Verification items for the finished model (mm, model axes). A direction names the side the tool comes from. Round coordinates to 2 decimals unless told otherwise and drop trailing zeros. Order: outer loops, then holes, each group sorted by start corner. A loop starts at its lowest first (then second) coordinate and runs counter-clockwise, first axis right, second up. Notation, with made-up numbers: M -20.75,-21 L 11.25,-21 A33 cw 11.25,8 Z; hole C -1,1.5 d4. An arc over 180 degrees is marked long. Use CSV: the item, a comma, the result in double quotes. Start each with the question number.
Q1. Sectioned sample at B-B (y = -9.5). Enter the section's corners in (x, z).
Q2. Set-up check for faces 1 (the face through (13, -15, -1.375)), 2 (the face through (13, -13.4, -4)), 3 (the face through (13, 0, 2)), 4 (the face through (-4, -3, -5)): record each of +Z, -Z, +X, -X, +Y, -Y from which the full face is reachable in a straight line by a thin tool's end or side.
Q3. Mould release check, pull along Y, two halves, no side actions. Record for faces 5 (the face through (-13.12, -14.784, -10.644)), 6 (the face through (0.195, 3.513, 11.032)), 7 (the face through (22.5, -3.8, -0.1)): +Y half, -Y half, draft (parallel to the pull), parting line (faces both ways), or undercut.
Q4. Scan lines: line 1 (X direction, y = 5, z = 10.25); line 2 (Y direction, x = -15, z = 10); line 3 (X direction, y = -3.5, z = -9). Record each from-to range of solid material in increasing order.
Q5. Gauge pin test, flat ends, axial feed: pin 1 Ø6 at (x, z) = (13, 7) entering from +Y; pin 2 Ø1.5 at (x, y) = (-7.5, -6) entering from -Z; pin 3 Ø4 at (x, y) = (15, 5) entering from -Z (3 decimals); pin 4 Ø14 at (y, z) = (-4.5, -3) entering from +X. Record the tip position at first contact, or that the pin passes through.
Q6. Sectioned sample at A-A (z = 1.5). Enter the section's corners in (x, y), and give its area (3 significant figures).
```python
from build123d import *

# Parameters (mm, degrees)
F0_W        = 45
F0_H        = 26.25
F1_DEPTH    = 17.4
F2_W        = 45
F2_H        = 4
F3_DEPTH    = 10
F5_DEPTH    = 45
F7_D        = 3
F8_T1_DEPTH = 112.5981529113
F9_W        = 8
F9_H        = 22.25
F9_H_2      = 1.1180170857
F10_DEPTH   = 21.5
F11_R       = 8.69999
F12_R       = 1


# Not quite as in the source:
# - a fillet or chamfer that OpenCascade refuses, or shapes differently, is made with other operations: its cross-section is extruded or revolved along the edge and cut away or added
# - a fillet or chamfer is up to 0.001 mm smaller than in the source, because OpenCascade refuses the exact size


with BuildPart() as f1:
    # F0 (on Front) → F1 (new body)
    with BuildSketch(Plane.XZ):
        Rectangle(F0_W, F0_H)
    extrude(amount=F1_DEPTH)

    # F2 (on face) → F3 (join)
    with BuildSketch(Plane(origin=(0, 0, 0), x_dir=(-1, 0, 0), z_dir=(0, 1, 0))):
        with Locations((0, 11.125)):
            Rectangle(F2_W, F2_H)
    extrude(amount=F3_DEPTH)

    # F4 (on face) → F5 (cut)
    with BuildSketch(Plane.YZ.offset(22.5)):
        with BuildLine():
            Line((-13.4, -1.375), (-13.4, -6.375))
            ThreePointArc((-13.4, -6.375), (-11.2118515201, -9.0669923606), (-8.1295833678, -7.475))
            Line((-8.1295833678, -7.475), (-4.5024615599, -7.475))
            Line((-4.5024615599, -7.475), (-4, -7.475))
            Line((-4, -7.475), (-4, 13.125))
            Line((-4, 13.125), (-17.4, 13.125))
            Line((-17.4, 13.125), (-17.4, -1.375))
            Line((-17.4, -1.375), (-13.4, -1.375))
        make_face()
    extrude(amount=-F5_DEPTH, mode=Mode.SUBTRACT)

    # F7 (through all)
    with Locations(Plane(origin=(0, 0, 9.125), x_dir=(1, 0, 0), z_dir=(0, 0, -1))):
        with Locations((-15, -5), (0, -5), (15, -5)):
            Hole(F7_D / 2)

    # F8: chamfer of 13 x 0.5 on 1 edges, made by hand

    # F8_s2 → F8_t1 (cut)
    with BuildSketch(Plane.YZ.offset(-56.2990764557)):
        Polygon((-3, 13.125), (10, 12.625), (10, 13.125), align=None)
    extrude(amount=F8_T1_DEPTH, mode=Mode.SUBTRACT)

    # F9 (on face) → F10 (cut)
    with BuildSketch(Plane(origin=(0, 0, 0), x_dir=(-1, 0, 0), z_dir=(0, 1, 0))):
        with Locations((0, -2)):
            Rectangle(F9_W, F9_H)
        with Locations((0, -13.6840085428)):
            Rectangle(F9_W, F9_H_2)
    extrude(amount=-F10_DEPTH, mode=Mode.SUBTRACT)

    # F11 (radius 8.7 in the source; OpenCascade refuses exactly that, so slightly less here)
    f11_edges = [f1.edges().sort_by_distance(p)[0] for p in [
        (-13.25, -17.4, -13.125),
        (-13.25, 0, -13.125),
        (13.25, -17.4, -13.125),
        (13.25, 0, -13.125),
    ]]
    fillet(f11_edges, radius=F11_R)

    # F12
    f12_edges = [f1.edges().sort_by_distance(p)[0] for p in [
        (0, 10, 9.125),
        (0, -4, 13.125),
    ]]
    fillet(f12_edges, radius=F12_R)


solid = f1.part
```
Verdict:
1,outline,"M -22.5,-13.09 L -4,-13.09 L -4,-8.87 L -22.5,-8.87 Z; M 4,-13.09 L 22.5,-13.09 L 22.5,-8.87 L 4,-8.87 Z"
2,face 1,"+Z, +X, -X, -Y"
2,face 2,"+Z, +X, -X"
2,face 3,"-Z, +X, -X, +Y"
2,face 4,"-Z, +Y, -Y"
3,face 5,"-Y half"
3,face 6,"undercut"
3,face 7,"draft"
4,line 1,"x = -22.5 to -16.5, -13.5 to -1.5, 1.5 to 13.5, 16.5 to 22.5"
4,line 2,"y = -4 to 3.5, 6.5 to 9.99"
4,line 3,"x = -22.5 to -4, 4 to 22.5"
5,pin 1,"stops at y = 9.99"
5,pin 2,"stops at z = -12.9"
5,pin 3,"stops at z = 9.125"
5,pin 4,"stops at x = 22.5"
6,outline,"M -22.5,-4 L -4,-4 L -4,0 L -22.5,0 Z; M 4,-4 L 22.5,-4 L 22.5,0 L 4,0 Z"
6,area,"148 mm²"
